from build123d import *

# Parameters (mm, degrees)
SKETCH005_W     = 9.5
SKETCH005_H     = 11.35
PAD002_DEPTH    = 2
SKETCH006_W     = 9.5
SKETCH006_H     = 1
POCKET_DEPTH    = 1
POCKET002_DEPTH = 0.5
FILLET008_R     = 0.25
FILLET009_R     = 0.1


with BuildPart() as part:
    # Sketch005 → Pad002 (new body)
    with BuildSketch(Plane.XY.offset(5.5)):
        with Locations((0, -0.825)):
            Rectangle(SKETCH005_W, SKETCH005_H)
    extrude(amount=PAD002_DEPTH)

    # Sketch006 → Pocket (cut)
    with BuildSketch(Plane(origin=(0, -6.5, 5.5), x_dir=(1, 0, 0), z_dir=(0, -1, 0))):
        with Locations((0, 0.5)):
            Rectangle(SKETCH006_W, SKETCH006_H)
    extrude(amount=-POCKET_DEPTH, mode=Mode.SUBTRACT)

    # Sketch008 → Pocket002 (cut)
    with BuildSketch(Plane.XY.offset(7.5)):
        with BuildLine():
            Line((4.75, 4.85), (2.5, 4.85))
            Line((2.5, 4.85), (2.5, 3.425))
            ThreePointArc((2.5, 3.425), (2.792893, 2.717893), (3.5, 2.425))
            Line((3.5, 2.425), (4.75, 2.425))
            Line((4.75, 2.425), (4.75, 4.85))
        make_face()
        with BuildLine():
            Line((-4.75, -6.5), (-2.5, -6.5))
            Line((-2.5, -6.5), (-2.5, -4.25))
            ThreePointArc((-2.5, -4.25), (-2.792893, -3.542893), (-3.5, -3.25))
            Line((-3.5, -3.25), (-4.75, -3.25))
            Line((-4.75, -3.25), (-4.75, -6.5))
        make_face()
    extrude(amount=-POCKET002_DEPTH, mode=Mode.SUBTRACT)

    # Fillet008
    fillet008_edges = [part.edges().sort_by_distance(p)[0] for p in [
        (-4.75, -6.5, 6.75),
        (4.75, -6.5, 7),
        (-4.75, 4.85, 6.5),
        (4.75, 4.85, 6.25),
    ]]
    fillet(fillet008_edges, radius=FILLET008_R)

    # Fillet009
    fillet009_edges = [part.edges().sort_by_distance(p)[0] for p in [
        (4.75, -1.9125, 7.5),
        (4.125, 2.425, 7.5),
        (2.5, 4.1375, 7.5),
        (-1, 4.85, 7.5),
        (-4.75, 0.675, 7.5),
        (-4.125, -3.25, 7.5),
        (-2.5, -5.375, 7.5),
        (1, -6.5, 7.5),
        (0, -6.5, 6.5),
        (-3.5, -6.5, 7),
        (-4.75, -4.75, 7),
        (3.5, 4.85, 7),
        (4.75, 3.5125, 7),
    ]]
    fillet(fillet009_edges, radius=FILLET009_R)


solid = part.part
Check sheet for the modelled part. Datum: model origin and axes. Units: mm. A direction names the side the tool comes from. Round coordinates to 2 decimals unless told otherwise and drop trailing zeros. Order: outer loops, then holes, each group sorted by start corner. A loop starts at its lowest first (then second) coordinate and runs counter-clockwise, first axis right, second up.
Q1. Depth check by flat-ended pin: P1, Ø0.6, axis at x = 4, y = 4, coming from the +Z side; P2, Ø0.7, axis at x = -0.5, y = -6, coming from the -Z side. Enter the tip coordinate at first touch or a pass-through.
Filled sheet:
P1: stops at z = 7
P2: stops at z = 6.5
Q2. Cross-section at B-B, the plane z = 6.3. Enter the section's corners in (x, y), plus the area to 3 significant figures.
Filled sheet:
outline: (-4.75, -5.5) - (4.75, -5.5) - (4.75, 4.6) arc R0.25 ccw to (4.5, 4.85) - (-4.5, 4.85) arc R0.25 ccw to (-4.75, 4.6) - close
area: 98.3 mm2
Q3. Set-up check for faces 1 (the face through (2.785, 2.726, 7.203)), 2 (the face through (0, -1, 7.5)), 3 (the face through (-2.785, -3.551, 7.203)), 4 (the face through (0, -6, 6.5)): record each of +Z, -Z, +X, -X, +Y, -Y from which the full face is reachable in a straight line by a thin tool's end or side.
Filled sheet:
face 1: +Z, +X, +Y
face 2: +Z, +X, -X, +Y, -Y
face 3: +Z, -X, -Y
face 4: -Z, +X, -X, -Y
Q4. Scan lines: L1, parallel to Y at x = 2.5, z = 6.4; L2, parallel to Z at x = 0, y = -6; L3, parallel to X at y = -5.5, z = 7.15. Record each from-to range of solid material in increasing order.
Filled sheet:
L1: y = -5.5 to 4.85
L2: z = 6.5 to 7.5
L3: x = -2.5 to 4.75
Q5. Cross-section at A-A, the plane x = -0.75. Enter the section's corners in (y, z).
Filled sheet:
outline: (-6.5, 6.6) arc R0.1 ccw to (-6.4, 6.5) - (-5.5, 6.5) - (-5.5, 5.5) - (4.85, 5.5) - (4.85, 7.4) arc R0.1 ccw to (4.75, 7.5) - (-6.4, 7.5) arc R0.1 ccw to (-6.5, 7.4) - close
